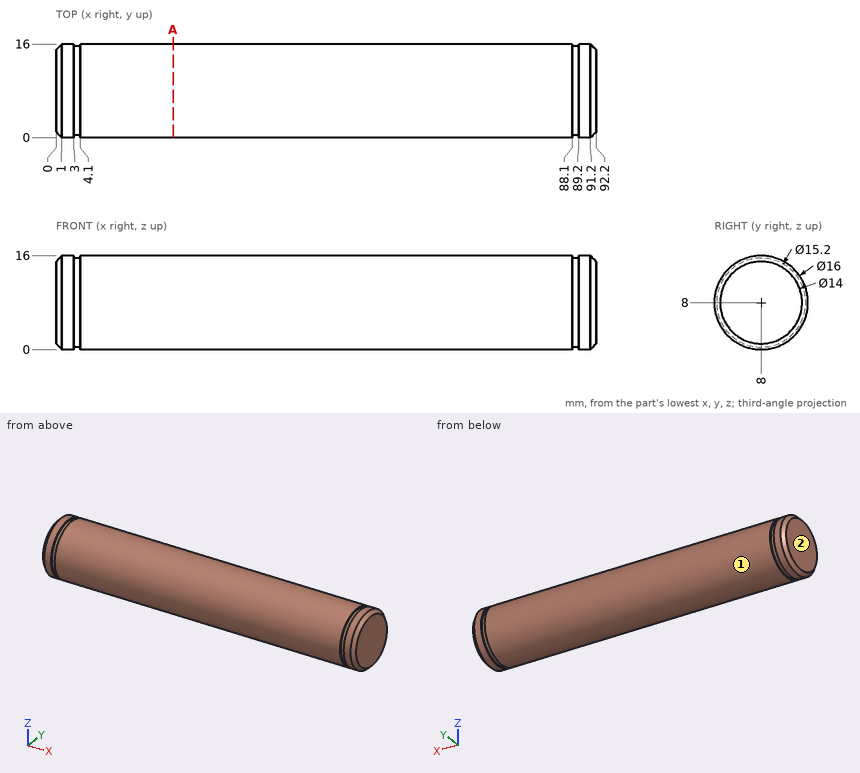
Print and shaded views of the part. All mm, measured from the part's lowest x, y and z. Coordinates: 2 decimals unless noted, no trailing zeros. Order: outer loops, then holes, each group sorted by start corner. A loop starts at its lowest first (then second) coordinate and runs counter-clockwise, first axis right, second up. Notation, with made-up numbers: (40.5, 1) - (56.5, 1) arc R21 ccw to (56.5, 32) - close; hole circle Ø9 at (44.5, 12.25). An arc over 180 degrees is marked (long way). Return JSON: item names as keys, results as strings. Group by question number.
Item 1: Pin check, flat tips, straight feed: pin 1 (2 mm diameter, centred on x = 18.5, z = 12.5, fed in from +Y); pin 2 (3 mm diameter, centred on x = 66, z = 10, fed in from -Y); pin 3 (4 mm diameter, centred on x = 74, z = 3.5, fed in from -Y). Stop position of each tip, or through.
Item 2: Cut at A-A (x = 20). List the corners of the cut face in (y, z).
Item 3: Pull direction Y, two halves, no side cores. Call the marked faces 1 and 2: pulls with the +Y half, pulls with the -Y half, needs draft (parallel to the pull), parting line crosses it, or undercut.
Item 4: Drill centre lines: probe 1 along Y at (x, z) = (19, 8.25); probe 2 along Y at (x, z) = (14, 10.5); probe 3 along Z at (x, y) = (81, 12.25). Where is each one in solid material? Low to high. Write a range as from..to.
Check values:
{
 "1": {"pin 1": "stops at y = 15.19", "pin 2": "stops at y = 0.02", "pin 3": "stops at y = 0.4"},
 "2": {"outline": "circle Ø16 at (8, 8)"},
 "3": {"face 1": "parting line crosses it", "face 2": "needs draft"},
 "4": {"probe 1": "y = 0..16", "probe 2": "y = 0.4..15.6", "probe 3": "z = 1.22..14.78"}
}
